Verification items for the finished model (mm, model axes). Coordinates: 2 decimals unless noted, no trailing zeros. Loops run counter-clockwise (first coordinate to the right, second up) from the corner with the lowest first, then second, coordinate; pieces in that order, holes last.
Q1. Sectioned sample at A-A (x = 0). Enter the section's corners in (y, z), then the cut area to 3 significant figures.
Q2. Go/stop test with flat-tipped pins: P1, Ø5, axis at x = 5.5, y = 4, coming from the -Z side; P2, Ø6, axis at x = 4.5, y = 5, coming from the +Z side; P3, Ø2, axis at y = 15.5, z = -2.5, coming from the +X side; P4, Ø8, axis at y = 21, z = 2.5, coming from the +X side. Record where each tip stops, or that it passes through.
Q3. Material ranges on probe 1 along X at (y, z) = (3.5, 5.25); probe 2 along X at (y, z) = (2.25, 4.5); probe 3 along Z at (x, y) = (-5, 16.5), recorded low to high.
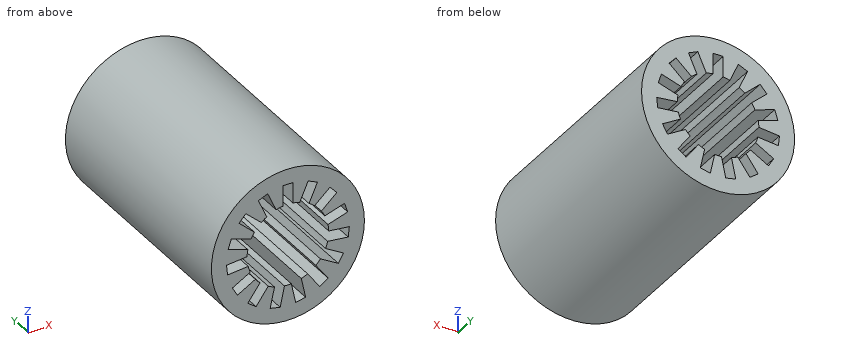
```python
from build123d import *

# Parameters (mm, degrees)
SKETCH1_R           = 7.5
BOSS_EXTRUDE1_DEPTH = 24


with BuildPart() as part:
    # Sketch1 → Boss-Extrude1 (new body)
    with BuildSketch(Plane(origin=(0, 0, 0), x_dir=(1, 0, 0), z_dir=(0, 1, 0))):
        Circle(SKETCH1_R)
        with BuildLine():
            Line((-0.5, -3.968626967), (-0.5, -6))
            Line((-0.5, -6), (0.5, -6))
            Line((0.5, -6), (0.5, -3.968626967))
            ThreePointArc((0.5, -3.968626967), (0.831646763, -3.912590403), (1.157413281, -3.82888946))
            Line((1.157413281, -3.82888946), (1.98364713, -5.684641067))
            Line((1.98364713, -5.684641067), (2.897192587, -5.277904424))
            Line((2.897192587, -5.277904424), (2.070958739, -3.422152817))
            ThreePointArc((2.070958739, -3.422152817), (2.351141009, -3.236067977), (2.614699291, -3.027102181))
            Line((2.614699291, -3.027102181), (4.12430365, -4.386356051))
            Line((4.12430365, -4.386356051), (4.793434256, -3.643211225))
            Line((4.793434256, -3.643211225), (3.283829898, -2.283957356))
            ThreePointArc((3.283829898, -2.283957356), (3.464101615, -2), (3.61988004, -1.701901435))
            Line((3.61988004, -1.701901435), (5.551830601, -2.329630224))
            Line((5.551830601, -2.329630224), (5.860847595, -1.378573708))
            Line((5.860847595, -1.378573708), (3.928897035, -0.750844919))
            ThreePointArc((3.928897035, -0.750844919), (3.978087581, -0.418113853), (3.999150644, -0.08242647))
            Line((3.999150644, -0.08242647), (6.019395604, 0.129909832))
            Line((6.019395604, 0.129909832), (5.914867141, 1.124431727))
            Line((5.914867141, 1.124431727), (3.894622181, 0.912095426))
            ThreePointArc((3.894622181, 0.912095426), (3.804226065, 1.236067977), (3.686931771, 1.551300781))
            Line((3.686931771, 1.551300781), (5.446152423, 2.566987298))
            Line((5.446152423, 2.566987298), (4.946152423, 3.433012702))
            Line((4.946152423, 3.433012702), (3.186931771, 2.417326185))
            ThreePointArc((3.186931771, 2.417326185), (2.972579302, 2.676522425), (2.7372089, 2.916794034))
            Line((2.7372089, 2.916794034), (3.931220011, 4.56020934))
            Line((3.931220011, 4.56020934), (3.122203017, 5.147994592))
            Line((3.122203017, 5.147994592), (1.928191906, 3.504579286))
            ThreePointArc((1.928191906, 3.504579286), (1.626946572, 3.654181831), (1.314197743, 3.7779471))
            Line((1.314197743, 3.7779471), (1.736543945, 5.764929759))
            Line((1.736543945, 5.764929759), (0.758396345, 5.97284145))
            Line((0.758396345, 5.97284145), (0.336050142, 3.985858791))
            ThreePointArc((0.336050142, 3.985858791), (0, 4), (-0.336050142, 3.985858791))
            Line((-0.336050142, 3.985858791), (-0.758396345, 5.97284145))
            Line((-0.758396345, 5.97284145), (-1.736543945, 5.764929759))
            Line((-1.736543945, 5.764929759), (-1.314197743, 3.7779471))
            ThreePointArc((-1.314197743, 3.7779471), (-1.626946572, 3.654181831), (-1.928191906, 3.504579286))
            Line((-1.928191906, 3.504579286), (-3.122203017, 5.147994592))
            Line((-3.122203017, 5.147994592), (-3.931220011, 4.56020934))
            Line((-3.931220011, 4.56020934), (-2.7372089, 2.916794034))
            ThreePointArc((-2.7372089, 2.916794034), (-2.972579302, 2.676522425), (-3.186931771, 2.417326185))
            Line((-3.186931771, 2.417326185), (-4.946152423, 3.433012702))
            Line((-4.946152423, 3.433012702), (-5.446152423, 2.566987298))
            Line((-5.446152423, 2.566987298), (-3.686931771, 1.551300781))
            ThreePointArc((-3.686931771, 1.551300781), (-3.804226065, 1.236067977), (-3.894622181, 0.912095426))
            Line((-3.894622181, 0.912095426), (-5.914867141, 1.124431727))
            Line((-5.914867141, 1.124431727), (-6.019395604, 0.129909832))
            Line((-6.019395604, 0.129909832), (-3.999150644, -0.08242647))
            ThreePointArc((-3.999150644, -0.08242647), (-3.978087581, -0.418113853), (-3.928897035, -0.750844919))
            Line((-3.928897035, -0.750844919), (-5.860847595, -1.378573708))
            Line((-5.860847595, -1.378573708), (-5.551830601, -2.329630224))
            Line((-5.551830601, -2.329630224), (-3.61988004, -1.701901435))
            ThreePointArc((-3.61988004, -1.701901435), (-3.464101615, -2), (-3.283829898, -2.283957356))
            Line((-3.283829898, -2.283957356), (-4.793434256, -3.643211225))
            Line((-4.793434256, -3.643211225), (-4.12430365, -4.386356051))
            Line((-4.12430365, -4.386356051), (-2.614699291, -3.027102181))
            ThreePointArc((-2.614699291, -3.027102181), (-2.351141009, -3.236067977), (-2.070958739, -3.422152817))
            Line((-2.070958739, -3.422152817), (-2.897192587, -5.277904424))
            Line((-2.897192587, -5.277904424), (-1.98364713, -5.684641067))
            Line((-1.98364713, -5.684641067), (-1.157413281, -3.82888946))
            ThreePointArc((-1.157413281, -3.82888946), (-0.831646763, -3.912590403), (-0.5, -3.968626967))
        make_face(mode=Mode.SUBTRACT)
    extrude(amount=BOSS_EXTRUDE1_DEPTH)


solid = part.part
```
Geometry check:
1. outline: (0, -7.5) - (24, -7.5) - (24, -4) - (0, -4) - close; (0, 6) - (24, 6) - (24, 7.5) - (0, 7.5) - close
1. area: 120 mm2
2. P1: stops at z = -6.87
2. P2: stops at z = 7.35
2. P3: stops at x = 7.35
2. P4: stops at x = 7.5
3. probe 1: x = -5.36 to -2.88, -1.79 to -0.5, 0.5 to 1.79, 2.88 to 5.36
3. probe 2: x = -6 to -2.55, -1.46 to -0.5, 0.5 to 1.46, 2.55 to 6
3. probe 3: z = -5.59 to -3.34, -2.31 to -1.03, -0.02 to 1.1, 2.15 to 5.59
